from build123d import *

# Parameters (mm, degrees)
PAD003_DEPTH = 2
FILLET_R     = 4


with BuildPart() as sphere:
    # Sphere → Sphere (revolve)
    with BuildSketch(Plane(origin=(8.5, 27.5, 11), x_dir=(1, 0, 0), z_dir=(0, -1, 0))):
        with BuildLine():
            ThreePointArc((0, -10), (10, 0), (0, 10))
            Line((0, 10), (0, -10))
        make_face()
    revolve(axis=Axis((8.5, 27.5, 11), (0, 0, 1)))


with BuildPart() as clone_of_countersunk002:
    # Sketch007 → Revolution001 (revolve)
    with BuildSketch(Plane.YZ):
        Polygon((3.2, 0), (1.5, -1.7), (1.5, -10), (0, -10), (0, 0), align=None)
    revolve(axis=Axis((0, 0, 0), (0, 0, 1)))


with BuildPart() as clone_of_countersunk002_1:
    # Clone005 placement: moved
    add(clone_of_countersunk002.part.moved(Location((17.5, 24.5, 2))))


with BuildPart() as obj1:
    # Sketch → Pad003 (new body)
    with BuildSketch(Plane.XY):
        with BuildLine():
            ThreePointArc((1.237539, 25.913851), (18.640493, 18.871057), (37.411488, 18.534097))
            ThreePointArc((37.411488, 18.534097), (39.499974, 20.988518), (37.43412, 23.462019))
            Line((27.412694, 25.229067), (37.43412, 23.462019))
            ThreePointArc((21.544649, 28.283778), (24.243589, 26.304833), (27.412694, 25.229067))
            Line((21.544649, 28.283778), (17.414214, 32.414214))
            ThreePointArc((17.414214, 32.414214), (16.765367, 32.847759), (16, 33))
            Line((16, 33), (3.428753, 33))
            ThreePointArc((3.428753, 33), (2.351121, 32.684847), (1.613108, 31.83871))
            ThreePointArc((1.613108, 31.83871), (0.872192, 29.955824), (0.353572, 28))
            ThreePointArc((0.353572, 28), (0.471658, 26.81968), (1.237539, 25.913851))
        make_face()
    extrude(amount=PAD003_DEPTH)

    # Cut003: cut Clone of Countersunk002
    add(clone_of_countersunk002_1.part, mode=Mode.SUBTRACT)

    # Cut004: cut Sphere
    add(sphere.part, mode=Mode.SUBTRACT)

    # Fillet
    fillet_edges = [obj1.edges().sort_by_distance(p)[0] for p in [
        (4.141101, 27.5, 2),
    ]]
    fillet(fillet_edges, radius=FILLET_R)


solid = obj1.part
Can you work these out from the model? Positions are in its coordinate system, mm. Coordinates: 2 decimals unless noted, no trailing zeros. Loops run counter-clockwise (first coordinate to the right, second up) from the corner with the lowest first, then second, coordinate; pieces in that order, holes last. Notation, with made-up numbers: (-8, -18) - (11, -18) arc R5 ccw to (11, -11) - close; hole circle Ø6 at (44, 7.5). An arc over 180 degrees is marked (long way). Answer as a JSON object with one key per item and string values. Group by question number.
Item 1: If we section it at A-A (x = 22.5): List the corners of the cut face in (y, z) for me.
Item 2: If I drill on L1, parallel to Y at x = 17.5, z = 0.25; L2, parallel to Y at x = 18, z = 1.15; L3, parallel to X at y = 32, z = 0.5, over which ranges is the centre line in solid material (lowest first)? Write a range as from..to.
Item 3: If we mould it in two halves opening along Y, with no side actions, what happens to faces 1 (the face through (39.5, 20.9, 1)), 2 (the face through (10, 33, 1)), 3 (the face through (18.41, 23.31, 0.15))? For each: released by +Y, released by -Y, zero draft, split by the parting line, or undercut.
Item 4: If we section it at B-B (x = 36): List the corners of the cut face in (y, z) for me, plus the area to 3 significant figures.
Item 5: For pin 1 (1.5 mm diameter, centred on x = 22.5, y = 29.5, fed in from +Z); pin 2 (1 mm diameter, centred on y = 24, z = 0.5, fed in from -X); pin 3 (1 mm diameter, centred on y = 22, z = 0.5, fed in from -X); pin 4 (4 mm diameter, centred on x = 17.5, y = 24.5, fed in from +Z), each with a flat end and sliding along its axis, tell me the tip position at first contact or that it passes through.
Returned:
{
 "1": {"outline": "(18.24, 0) - (27.43, 0) - (27.43, 2) - (18.24, 2) - close"},
 "2": {"L1": "y = 19.12..23, 26..32.33", "L2": "y = 19.01..22.2, 26.8..31.83", "L3": "x = 1.7..17.83"},
 "3": {"face 1": "split by the parting line", "face 2": "released by +Y", "face 3": "undercut"},
 "4": {"outline": "(18.32, 0) - (23.71, 0) - (23.71, 2) - (18.32, 2) - close", "area": "10.8 mm²"},
 "5": {"pin 1": "passes through", "pin 2": "stops at x = 3.59", "pin 3": "stops at x = 7.51", "pin 4": "stops at z = 0.8"}
}
